Drawing for the job (mm, zero at the part's lowest x, y, z). A direction names the side the tool comes from. Round coordinates to 2 decimals unless told otherwise and drop trailing zeros. Loops run counter-clockwise (first coordinate to the right, second up) from the corner with the lowest first, then second, coordinate; pieces in that order, holes last. Notation, with made-up numbers: (3.5, 71.5) -> (53.5, 71.5) arc R31 ccw to (53.5, 96.5) -> close; hole circle Ø4 at (80, -27.75). An arc over 180 degrees is marked (long way). Put each result on its own line as item: value. Start each with the question number.
Item 1: Cut at A-A, the plane x = 7.5. List the corners of the cut face in (y, z), plus the area to 4 significant figures.
Item 2: Cut at D-D, the plane y = 4.25. List the corners of the cut face in (x, z).
Item 3: Flat gauge pins, fed straight in: pin 1 Ø4.5 at (x, z) = (7.5, 7.5) entering from +Y; pin 2 Ø1.5 at (y, z) = (1.5, 12) entering from -X. Where does each tip first touch, or does it go through?
Item 4: Tool access for the marked faces 1 and 2: list every direction of +Z, -Z, +X, -X, +Y, -Y with a clear straight run to the whole face (end or side of a thin tool).
Item 5: Cut at C-C, the plane z = 1.5. List the corners of the cut face in (x, y).
Item 6: Drill centre lines: probe 1 along X at (y, z) = (2.95, 7.5); probe 2 along Y at (x, z) = (4.5, 14); probe 3 along X at (y, z) = (3.15, 8.75). Where is each one in solid material? Low to high. Write a range as [from, to].
Item 7: Cut at B-B, the plane z = 7.5. List the corners of the cut face in (x, y), plus the area to 4 significant figures.
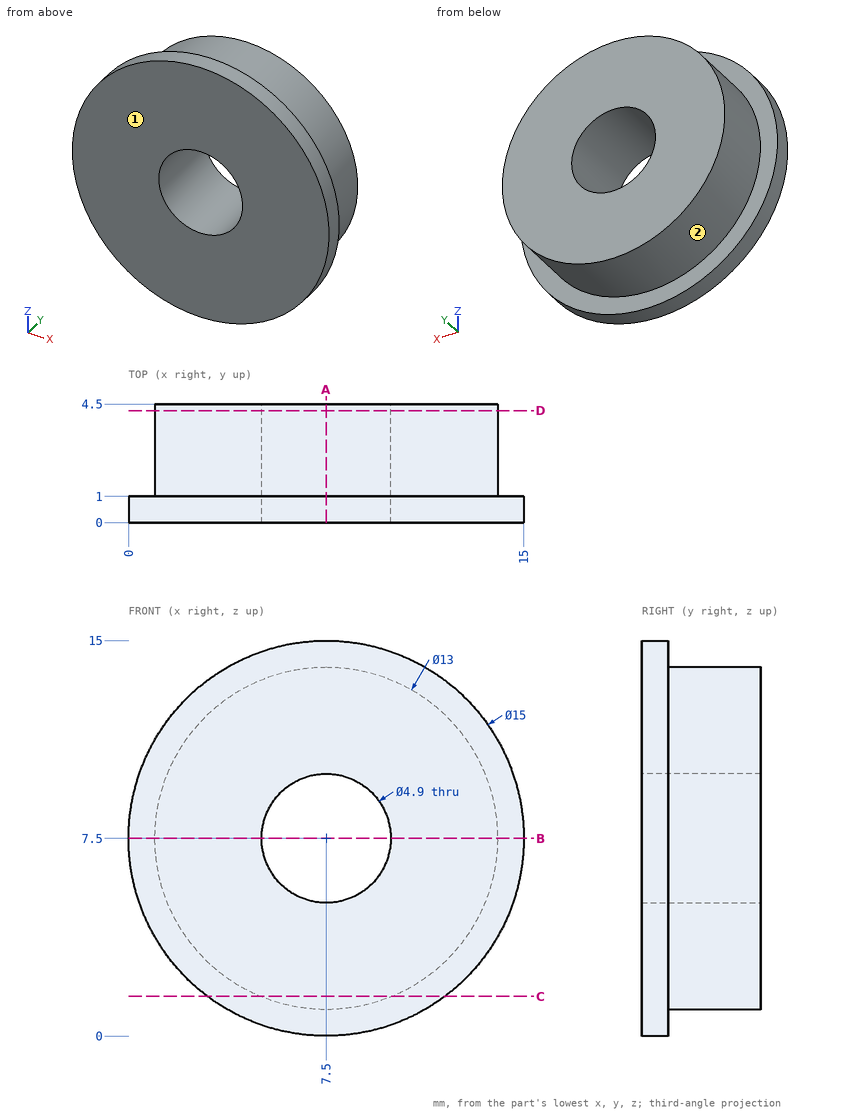
Reply:
1. outline: (0, 0) -> (1, 0) -> (1, 1) -> (4.5, 1) -> (4.5, 5.05) -> (0, 5.05) -> close; (0, 9.95) -> (4.5, 9.95) -> (4.5, 14) -> (1, 14) -> (1, 15) -> (0, 15) -> close
1. area: 38.45 mm^2
2. outline: circle Ø13 at (7.5, 7.5); hole circle Ø4.9 at (7.5, 7.5)
3. pin 1: passes through
3. pin 2: stops at x = 1.12
4. face 1: +Z, -Z, +X, -X, -Y
4. face 2: +Y
5. outline: (3, 0) -> (12, 0) -> (12, 1) -> (10, 1) -> (10, 4.5) -> (5, 4.5) -> (5, 1) -> (3, 1) -> close
6. probe 1: x = [1, 5.05], [9.95, 14]
6. probe 2: y = [0, 1]
6. probe 3: x = [1.12, 5.39], [9.61, 13.88]
7. outline: (0, 0) -> (5.05, 0) -> (5.05, 4.5) -> (1, 4.5) -> (1, 1) -> (0, 1) -> close; (9.95, 0) -> (15, 0) -> (15, 1) -> (14, 1) -> (14, 4.5) -> (9.95, 4.5) -> close
7. area: 38.45 mm^2
